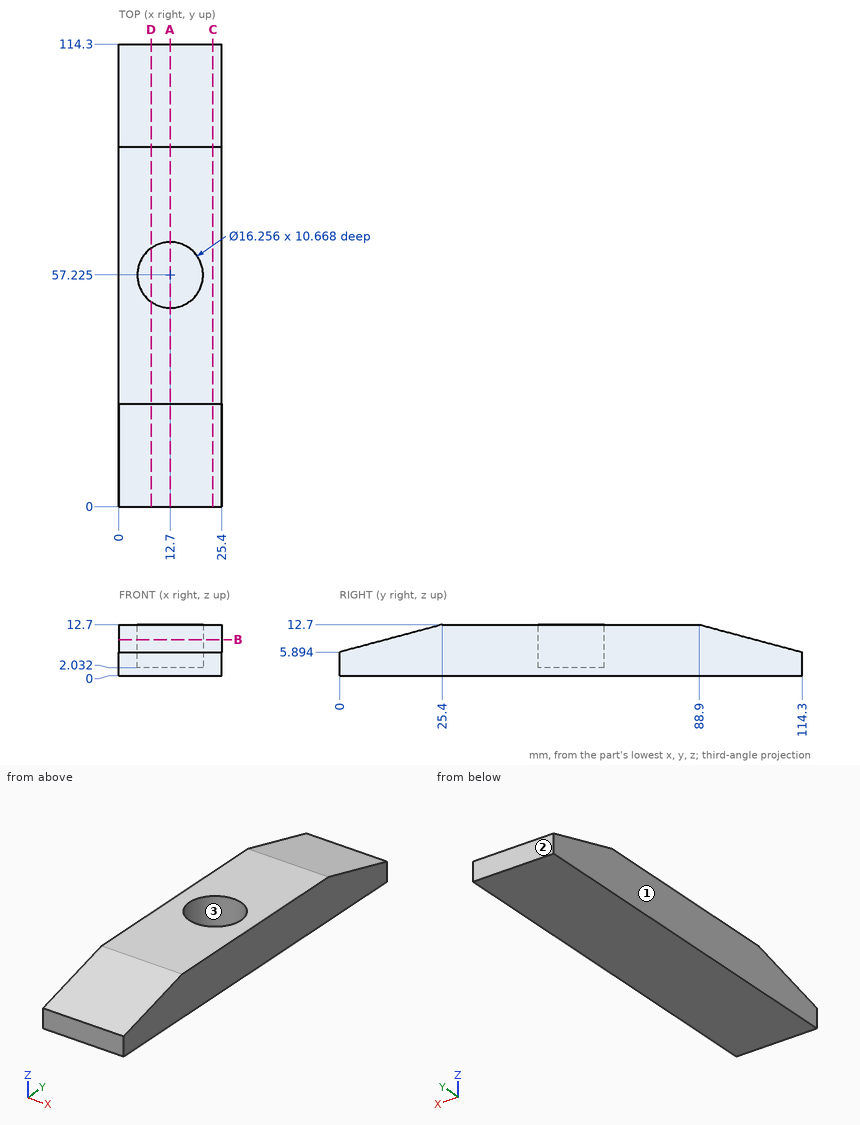
Geometry: see drawing. Coordinates: mm, zero at the bounding-box minimum. Round coordinates to 2 decimals unless told otherwise and drop trailing zeros. Loops run counter-clockwise (first coordinate to the right, second up) from the corner with the lowest first, then second, coordinate; pieces in that order, holes last. Notation, with made-up numbers: (49, 88) - (99, 88) arc R26 ccw to (99, 122) - close; hole circle Ø7 at (-8, 10.25). An arc over 180 degrees is marked (long way). Write item = value, one per line. Start each with the question number.
(1) Pin query (flat end, axial travel): pin 1 (5 mm diameter, centred on x = 13, y = 55, fed in from +Z); pin 2 (4 mm diameter, centred on x = 11, y = 11.5, fed in from +Z). Return the tip coordinate at first contact, or that it passes through.
(2) Section query A-A, the plane x = 12.7. Output: boundary loops of the cut face in (y, z), plus the area to 3 significant figures.
(3) Section query C-C, the plane x = 23.25. Output: boundary loops of the cut face in (y, z), plus the area to 3 significant figures.
(4) Section query D-D, the plane x = 8. Output: boundary loops of the cut face in (y, z).
(5) Section query B-B, the plane z = 9. Output: boundary loops of the cut face in (x, y) (1 decimal).
(6) Pull-direction query (Y, two-part tool) for the marked faces 1, 2 and 3; classes: +Y half, -Y half, draft (parallel to the pull), parting line (faces both ways), or undercut.
(7) Ray query, line 1 along X through (y, z) = (58, 11); line 2 along Y through (x, z) = (12.7, 4.75); line 3 along X through (y, z) = (63, 7). Return the intervals inside material, ascending. Write a range as from..to.
Conclusion:
q1.pin_1 = 2.03
q1.pin_2 = 9.51
q2.outline = (0, 0) - (114.3, 0) - (114.3, 5.89) - (88.9, 12.7) - (65.35, 12.7) - (65.35, 2.03) - (49.1, 2.03) - (49.1, 12.7) - (25.4, 12.7) - (0, 5.89) - close
q2.area = 1,110 mm2
q3.outline = (0, 0) - (114.3, 0) - (114.3, 5.89) - (88.9, 12.7) - (25.4, 12.7) - (0, 5.89) - close
q3.area = 1,280 mm2
q4.outline = (0, 0) - (114.3, 0) - (114.3, 5.89) - (88.9, 12.7) - (63.86, 12.7) - (63.86, 2.03) - (50.59, 2.03) - (50.59, 12.7) - (25.4, 12.7) - (0, 5.89) - close
q5.outline = (0, 11.6) - (25.4, 11.6) - (25.4, 102.7) - (0, 102.7) - close; hole circle Ø16.3 at (12.7, 57.2)
q6.face_1 = draft
q6.face_2 = +Y half
q6.face_3 = undercut
q7.line_1 = 0..4.61, 20.79..25.4
q7.line_2 = 0..49.1, 65.35..114.3
q7.line_3 = 0..6.98, 18.42..25.4
